```python
from build123d import *

# Parameters (mm, degrees)
SKETCH_1_W                  = 25
SKETCH_1_H                  = 40
EXTRUDE_1_DEPTH             = 25
SKETCH_2_W                  = 22
SKETCH_2_H                  = 22
CUT_EXTRUDE_1_DEPTH         = 74.239333694
HOLE_WIZARD_4_2_4_2_1_D     = 4.2
HOLE_WIZARD_4_2_4_2_1_DEPTH = 25
HOLE_WIZARD_4_2_4_2_2_D     = 4.2


with BuildPart() as part:
    # 草图1 → 凸台-拉伸1 (new body)
    with BuildSketch(Plane.XY.offset(20)):
        with Locations((45.5, 200)):
            Rectangle(SKETCH_1_W, SKETCH_1_H)
    extrude(amount=-EXTRUDE_1_DEPTH)

    # 草图2 → 切除-拉伸1 (cut, through all)
    with BuildSketch(Plane(origin=(0, 220, 0), x_dir=(-1, 0, 0), z_dir=(0, 1, 0))):
        with Locations((-47, 9)):
            Rectangle(SKETCH_2_W, SKETCH_2_H)
    extrude(amount=-CUT_EXTRUDE_1_DEPTH, mode=Mode.SUBTRACT)

    # Ø4.2 (4.2) 直径孔1
    with Locations(Plane(origin=(0, 0, -5), x_dir=(-1, 0, 0), z_dir=(0, 0, -1))):
        with Locations((-48, 185), (-48, 215)):
            Hole(HOLE_WIZARD_4_2_4_2_1_D / 2, depth=HOLE_WIZARD_4_2_4_2_1_DEPTH)

    # Ø4.2 (4.2) 直径孔2 (through all)
    with Locations(Plane(origin=(36, 0, 0), x_dir=(0, 0, -1), z_dir=(1, 0, 0))):
        with Locations((-10, 185), (-10, 215), (-5, 200), (-15, 200)):
            Hole(HOLE_WIZARD_4_2_4_2_2_D / 2)


solid = part.part
```
Can you work these out from the model? Positions are in its coordinate system, mm. A direction names the side the tool comes from. Give positions to 0.01 mm unless a question says otherwise; leave off trailing zeros. Order: outer loops, then holes, each group sorted by start corner. A loop starts at its lowest first (then second) coordinate and runs counter-clockwise, first axis right, second up. Notation, with made-up numbers: (68.25, 19.25) - (100.25, 19.25) arc R10 cw to (100.25, 30.25) - close; hole circle Ø7 at (73, -23). An arc over 180 degrees is marked (long way). Use a Markdown table: item, result. Add a question column.
Q1. Please list where these lines run through material, in increasing order: line 1 along Y through (x, z) = (48, -3.9); line 2 along Z through (x, y) = (34.4, 185); line 3 along Z through (x, y) = (42.75, 189).
Q2. I'm going to push flat-ended pins straight in: pin 1 (6.5 mm diameter, centred on y = 200, z = 5, fed in from +X); pin 2 (6.5 mm diameter, centred on x = 45, y = 206.5, fed in from +Z). Where does each tip first touch, or does it pass through?
Q3. If we section it at A-A on x = 48: Write out the boundary of the cut face in (y, z), plus the area to 3 significant figures.
Q4. If we section it at B-B on z = 15: Write out the boundary of the cut face in (x, y), plus the area to 3 significant figures.
Q5. On a 3-axis mill with a long thin cutter (end or side, diameter ignored), from which of +Z, -Z, +X, -X, +Y, -Y can I reach the whole of each face in a straight line? I mean faces 1 (the flat face through (33, 200, 8)), 2 (the flat face through (36, 200, 9)). Say none if no direction works.
Q6. If we section it at D-D on z = 9: Write out the boundary of the cut face in (x, y), plus the area to 3 significant figures.
Q7. If we section it at C-C on y = 199.5: Write out the boundary of the cut face in (x, z), plus the area to 3 significant figures.
Q8. If we mould it in two halves opening along X, with no side actions, what happens to faces 3 (the cylindrical face through (47.727, 217.082, -3.479)), 4 (the flat face through (34, 200, 20)), 5 (the flat face through (58, 200, -3))? For each: released by +X, released by -X, zero draft, split by the parting line, or undercut.
Answers follow:
| question | item | result |
|---|---|---|
| 1 | line 1 | y = 180 to 182.9, 187.1 to 212.9, 217.1 to 220 |
| 1 | line 2 | z = -5 to 7.9, 12.1 to 20 |
| 1 | line 3 | z = -5 to -2 |
| 2 | pin 1 | stops at x = 36 |
| 2 | pin 2 | stops at z = -2 |
| 3 | outline | (180, -5) - (182.9, -5) - (182.9, -2) - (180, -2) - close; (187.1, -5) - (212.9, -5) - (212.9, -2) - (187.1, -2) - close; (217.1, -5) - (220, -5) - (220, -2) - (217.1, -2) - close |
| 3 | area | 94.8 mm^2 |
| 4 | outline | (33, 180) - (36, 180) - (36, 197.9) - (33, 197.9) - close; (33, 202.1) - (36, 202.1) - (36, 220) - (33, 220) - close |
| 4 | area | 107 mm^2 |
| 5 | face 1 | +Z, -Z, -X, +Y, -Y |
| 5 | face 2 | +Z, +X, +Y, -Y |
| 6 | outline | (33, 180) - (36, 180) - (36, 183.15) - (33, 183.15) - close; (33, 186.85) - (36, 186.85) - (36, 213.15) - (33, 213.15) - close; (33, 216.85) - (36, 216.85) - (36, 220) - (33, 220) - close |
| 6 | area | 97.8 mm^2 |
| 7 | outline | (33, -5) - (58, -5) - (58, -2) - (36, -2) - (36, 2.96) - (33, 2.96) - close; (33, 7.04) - (36, 7.04) - (36, 12.96) - (33, 12.96) - close; (33, 17.04) - (36, 17.04) - (36, 20) - (33, 20) - close |
| 7 | area | 117 mm^2 |
| 8 | face 3 | undercut |
| 8 | face 4 | zero draft |
| 8 | face 5 | released by +X |
